Geometry: final body of the model. Coordinates: model frame, mm. Coordinates: 2 decimals unless noted, no trailing zeros. Write each loop counter-clockwise with the first axis right and the second up, starting at its lowest first coordinate (ties: lowest second). Pieces come first, ordered by that corner, then holes.
from build123d import *


# Not quite as in the source:
# - a fillet or chamfer that OpenCascade refuses, or shapes differently, is made with other operations: its cross-section is extruded or revolved along the edge and cut away or added


with BuildPart() as f1:
    # F0 (on Front) → F1 (revolve)
    with BuildSketch(Plane.XZ):
        with BuildLine():
            Line((0, 7.1883308701), (0, -30.2243120968))
            Line((0, -30.2243120968), (10.8706858009, -30.2243120968))
            ThreePointArc((10.8706858009, -30.2243120968), (9.889180772, -29.2428070679), (10.8706858009, -28.261302039))
            Line((10.8706858009, -28.261302039), (9.4850324094, -26.413762942))
            Line((9.4850324094, -26.413762942), (9.4850324094, -25.1435805112))
            ThreePointArc((9.4850324094, -25.1435805112), (6.1587538552, -12.5717902556), (9.4850324094, 0))
            Line((9.4850324094, 0), (13.0181515325, 6.2093746912))
            Line((13.0181515325, 6.2093746912), (7.0601375774, 2.4540154263))
            Line((7.0601375774, 2.4540154263), (4.3007276076, 6.8319196288))
            Line((4.3007276076, 6.8319196288), (2.7877071407, 3.1468416564))
            Line((2.7877071407, 3.1468416564), (0, 7.1883308701))
        make_face()
    revolve(axis=Axis((0, 0, -11.5179906134), (0, 0, -1)))

    # F2: fillet of radius 5.08 on 3 edges, made by hand

    # F2_s1 → F2_t2 (revolve, cut)
    with BuildSketch(Plane.XZ):
        with BuildLine():
            ThreePointArc((9.8965199445, -29.1230030365), (9.8769062732, -27.7401129903), (9.4850324094, -26.413762942))
            Line((9.4850324094, -26.413762942), (9.577642948, -26.3719795942))
            ThreePointArc((9.577642948, -26.3719795942), (10.2591391248, -27.2765725167), (10.9519658206, -28.2003420652))
            Line((10.9519658206, -28.2003420652), (10.8706858009, -28.362902039))
            ThreePointArc((10.8706858009, -28.362902039), (10.2877069025, -28.5837407102), (9.9973602337, -29.1354044906))
            Line((9.9973602337, -29.1354044906), (9.8965199445, -29.1230030365))
        make_face()
    revolve(axis=Axis((0, 0, -28.261302039), (0, 0, -1)), mode=Mode.SUBTRACT)

    # F2_s3 → F2_t4 (revolve, cut)
    with BuildSketch(Plane.XZ):
        with BuildLine():
            ThreePointArc((9.4850324094, -26.413762942), (9.3435632486, -25.2320724327), (8.9310390894, -24.1157258013))
            Line((8.9310390894, -24.1157258013), (9.0215590688, -24.0695880366))
            ThreePointArc((9.0215590688, -24.0695880366), (9.2915699789, -24.584629862), (9.5733382381, -25.0933347091))
            Line((9.5733382381, -25.0933347091), (9.5866324094, -25.1435805112))
            Line((9.5866324094, -25.1435805112), (9.5866322552, -26.4135859201))
            Line((9.5866322552, -26.4135859201), (9.4850324094, -26.413762942))
        make_face()
    revolve(axis=Axis((0, 0, -25.1435805112), (0, 0, -1)), mode=Mode.SUBTRACT)


solid = f1.part
Item 1: Pull-direction query (Y, two-part tool) for faces 1 (the conical face through (-3.52, 2.7, 6.62)), 2 (the flat face through (0, 0, -30.224)), 3 (the conical face through (2.89, -0.91, 3.74)), 4 (the conical face through (-2.104, 9.475, 0.388)); classes: released by +Y, released by -Y, zero draft, split by the parting line, or undercut.
Derived:
face 1: undercut
face 2: zero draft
face 3: undercut
face 4: split by the parting line
Item 2: Material intervals for probe 1 along Y at (x, z) = (5.5, 3.5); probe 2 along Z at (x, y) = (4.75, 6.25); probe 3 along Z at (x, y) = (7, -3.5), sorted ascending.
Derived:
probe 1: y = -10.07 to -6.77, -3.27 to 3.27, 6.77 to 10.07
probe 2: z = -30.22 to -21.69, -3.45 to 2.95
probe 3: z = -30.22 to -21.63, -3.52 to 2.94
Item 3: Pin query (flat end, axial travel): pin 1 (2 mm diameter, centred on x = -0.5, z = -23.5, fed in from +Y); pin 2 (12 mm diameter, centred on x = -3, y = -9.5, fed in from +Z); pin 3 (10 mm diameter, centred on y = -8.5, z = -20, fed in from -X). Return the tip coordinate at first contact, or that it passes through.
Derived:
pin 1: stops at y = 9.1
pin 2: stops at z = 6.83
pin 3: stops at x = -7.09
Item 4: Section A-A, the plane z = 4. Output: boundary loops of the cut face in (x, y), plus the area to 3 significant figures.
Derived:
outline: circle Ø23.52 at (0, 0); circle Ø12.17 at (0, 0); circle Ø4.4 at (0, 0); hole circle Ø19.03 at (0, 0); hole circle Ø6.28 at (0, 0)
area: 251 mm2
Item 5: Section C-C, the plane z = -13. Output: boundary loops of the cut face in (x, y), plus the area to 3 significant figures.
Derived:
outline: circle Ø12.32 at (0, 0)
area: 119 mm2
Item 6: Section B-B, the plane z = -22. Output: boundary loops of the cut face in (x, y).
Derived:
outline: circle Ø15.94 at (0, 0)
